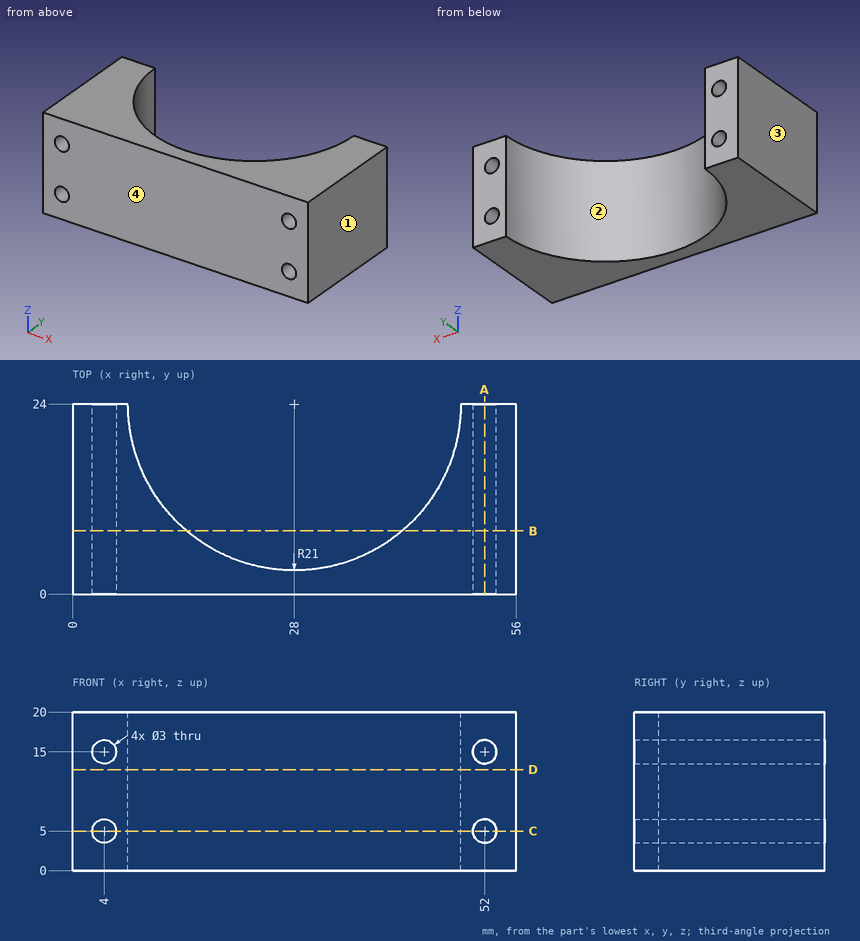
Source: three-view drawing plus pictorial views. Frame: mm from the lowest corner of the part. Round coordinates to 2 decimals unless told otherwise and drop trailing zeros. Write each loop counter-clockwise with the first axis right and the second up, starting at its lowest first coordinate (ties: lowest second). Pieces come first, ordered by that corner, then holes. Notation, with made-up numbers: (-4.75, -36) -> (16.25, -36) arc R18 cw to (16.25, -12) -> close; hole circle Ø11 at (78, -7). An arc over 180 degrees is marked (long way). Return JSON: item names as keys, results as strings.
Q1. Mould query, pull axis X, two halves, no side actions, for the marked faces 1, 2, 3 and 4. Classes: +X half, -X half, draft (parallel to the pull), parting line (faces both ways), or undercut.
From the geometry:
{"face 1": "+X half", "face 2": "undercut", "face 3": "-X half", "face 4": "draft"}
Q2. Ray query, line 1 (Z direction, x = 52, y = 14.25); line 2 (X direction, y = 17.75, z = 15); line 3 (X direction, y = 15.5, z = 4.5). Return the intervals inside material, ascending.
From the geometry:
{"line 1": "0 to 3.5, 6.5 to 13.5, 16.5 to 20", "line 2": "0 to 2.5, 5.5 to 7.95, 48.05 to 50.5, 53.5 to 56", "line 3": "0 to 2.59, 5.41 to 8.8, 47.2 to 50.59, 53.41 to 56"}
Q3. Section B-B on y = 8. Return the cut outline in (x, z), and give its area (3 significant figures).
From the geometry:
{"outline": "(0, 0) -> (14.4, 0) -> (14.4, 20) -> (0, 20) -> close; (41.6, 0) -> (56, 0) -> (56, 20) -> (41.6, 20) -> close; hole circle Ø3 at (4, 5); hole circle Ø3 at (4, 15); hole circle Ø3 at (52, 5); hole circle Ø3 at (52, 15)", "area": "548 mm2"}
Q4. Section D-D on z = 12.75. Return the cut outline in (x, y), and give its area (3 significant figures).
From the geometry:
{"outline": "(0, 0) -> (56, 0) -> (56, 24) -> (49, 24) arc R21 cw to (7, 24) -> (0, 24) -> close", "area": "651 mm2"}
Q5. Section C-C on z = 5. Return the cut outline in (x, y).
From the geometry:
{"outline": "(0, 0) -> (2.5, 0) -> (2.5, 24) -> (0, 24) -> close; (5.5, 0) -> (50.5, 0) -> (50.5, 24) -> (49, 24) arc R21 cw to (7, 24) -> (5.5, 24) -> close; (53.5, 0) -> (56, 0) -> (56, 24) -> (53.5, 24) -> close"}
Q6. First-contact query: pin 1 Ø1.5 at (x, z) = (24.5, 8) entering from +Y; pin 2 Ø2.5 at (x, z) = (52, 5) entering from +Y. Flat tips, straight axial feed; report the tip coordinate or a pass-through.
From the geometry:
{"pin 1": "y = 3.43", "pin 2": "through"}
Q7. Section A-A on x = 52. Return the cut outline in (y, z).
From the geometry:
{"outline": "(0, 0) -> (24, 0) -> (24, 3.5) -> (0, 3.5) -> close; (0, 6.5) -> (24, 6.5) -> (24, 13.5) -> (0, 13.5) -> close; (0, 16.5) -> (24, 16.5) -> (24, 20) -> (0, 20) -> close"}
